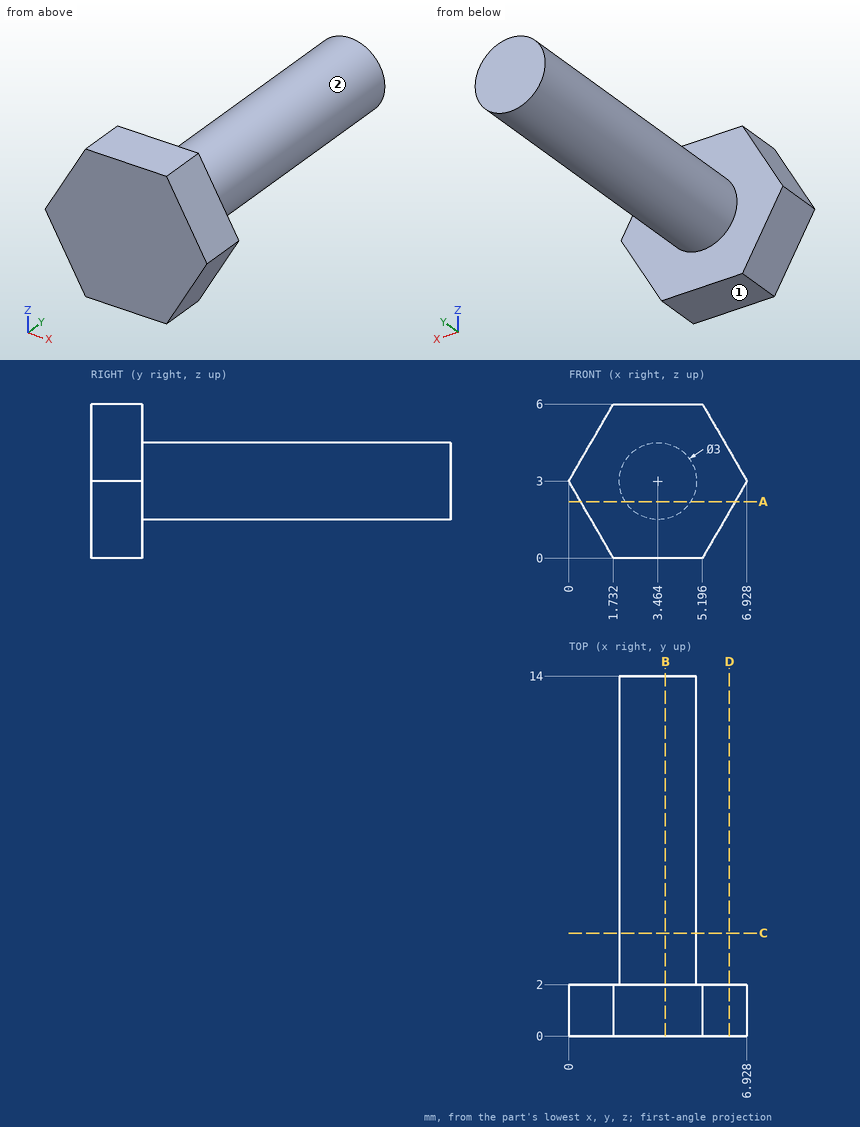
Verification items for this drawing (mm, ordinates from the low corner). A direction names the side the tool comes from. Round coordinates to 2 decimals unless told otherwise and drop trailing zeros. Write each loop counter-clockwise with the first axis right and the second up, starting at its lowest first coordinate (ties: lowest second). Pieces come first, ordered by that corner, then holes. Notation, with made-up numbers: M 77.25,24.5 L 136.25,24.5 A14 cw 136.25,49.5 Z; hole C 2,58 d6. An arc over 180 degrees is marked long. Write item = value, one per line. Start each with the question number.
1. Section check B-B, the plane x = 3.75. Record the cut outline in (y, z).
2. Gauge pin test, flat ends, axial feed: pin 1 (1 mm diameter, centred on y = 5.5, z = 3.5, fed in from -X); pin 2 (3 mm diameter, centred on x = 3, y = 8, fed in from +Z); pin 3 (2 mm diameter, centred on y = 1.5, z = 1.5, fed in from +X). Record the tip position at first contact, or that the pin passes through.
3. Scan lines: line 1 (Y direction, x = 5, z = 2.5); line 2 (X direction, y = 10.75, z = 2.95) (1 decimal); line 3 (X direction, y = 4.75, z = 3.65). Record each from-to range of solid material in increasing order. Write a range as [from, to].
4. Section check C-C, the plane y = 4. Record the cut outline in (x, z).
5. Section check D-D, the plane x = 6.25. Record the cut outline in (y, z) (1 decimal).
6. Section check A-A, the plane z = 2.2. Record the cut outline in (x, y) (1 decimal).
7. Tool access check on the marked faces 1 and 2. Record the directions out of +Z, -Z, +X, -X, +Y, -Y that give a thin tool (end or side, any length) a straight path to the whole face; none if there is none.
Results found:
q1.outline = M 0,0 L 2,0 L 2,1.53 L 14,1.53 L 14,4.47 L 2,4.47 L 2,6 L 0,6 Z
q2.pin_1 = 1.96
q2.pin_2 = 4.5
q2.pin_3 = 6.64
q3.line_1 = [0, 2]
q3.line_2 = [2, 5]
q3.line_3 = [2.11, 4.82]
q4.outline = C 3.46,3 d3
q5.outline = M 0,1.8 L 2,1.8 L 2,4.2 L 0,4.2 Z
q6.outline = M 0.5,0 L 6.5,0 L 6.5,2 L 4.7,2 L 4.7,14 L 2.2,14 L 2.2,2 L 0.5,2 Z
q7.face_1 = -Z, +X, -X, +Y, -Y
q7.face_2 = +Y
